Read the model definition and answer for the solid it produces. Units are mm, in the model's axes. A direction names the side the tool comes from. Round coordinates to 2 decimals unless told otherwise and drop trailing zeros. Order: outer loops, then holes, each group sorted by start corner. A loop starts at its lowest first (then second) coordinate and runs counter-clockwise, first axis right, second up. Notation, with made-up numbers: (24.25, -7) - (64.25, -7) arc R16 cw to (64.25, 6) - close; hole circle Ø1 at (80, -20.5). An arc over 180 degrees is marked (long way). Put each result on its own line as item: value. Start each with the question number.
Q1. Section C-C on x = -27.94 is taken. Give the vertices of the cut face in (y, z) (3 decimals).
Q2. Which of the six approach directions +Z, -Z, +X, -X, +Y, -Y give full straight-line access (tool end or side, diameter ignored) to faces 1 (the face through (-31.75, 4, 0)), 2 (the face through (0, 6.35, 0))?
Q3. Section A-A on z = -27.94 is taken. Give the vertices of the cut face in (x, y) (3 decimals).
Q4. For a pull along Z with two mould halves and no side action, classify faces 3 (the face through (-29.44, 3.88, -28.01)), 4 (the face through (14, 0, 0)), 5 (the face through (0, 4, -31.75)) as pulls with the +Z half, pulls with the -Z half, needs draft (parallel to the pull), parting line crosses it, or undercut.
Q5. This flat-tipped pin is pushed along its axis until it touches: pin 1 Ø7.5 at (x, z) = (-1.5, -3) entering from -Y. Where does it stop, or does it pass through?
Q6. Section D-D on z = 0 is taken. Give the vertices of the cut face in (x, y).
Q7. Find the intervals of material crossed by line 1 along X through (y, z) = (4, -27.94); line 2 along Z through (x, y) = (0, 4), in increasing order. Write a range as from..to.
Q8. Section B-B on y = 2 is taken. Give the vertices of the cut face in (x, z), then the cut area to 3 significant figures.
from build123d import *

# Parameters (mm, degrees)
SKETCH1_W                       = 63.5
SKETCH1_H                       = 63.5
BOSS_EXTRUDE1_DEPTH             = 7.62
F_3_0MM_DOWEL_HOLE1_D           = 3
F_3_0MM_DOWEL_HOLE1_DEPTH       = 7.62
F_3_0MM_DOWEL_HOLE1_CSINK_D     = 3.05
F_3_0MM_DOWEL_HOLE1_CSINK_ANGLE = 90
LPATTERN1_COUNT                 = 2
LPATTERN1_PITCH                 = 55.88
LPATTERN1_COUNT_DIR2            = 2
LPATTERN1_PITCH_DIR2            = 55.88
SKETCH6_R                       = 12.7
CUT_EXTRUDE1_DEPTH              = 6.35


with BuildPart() as part:
    # Sketch1 → Boss-Extrude1 (new body)
    with BuildSketch(Plane(origin=(0, 0, 0), x_dir=(1, 0, 0), z_dir=(0, 1, 0))):
        Rectangle(SKETCH1_W, SKETCH1_H)
    extrude(amount=BOSS_EXTRUDE1_DEPTH)

    # Ø3.0mm Dowel Hole1
    with Locations(Plane(origin=(0, 0, 0), x_dir=(-1, 0, 0), z_dir=(0, -1, 0))):
        with Locations((-27.94, -27.94)):
            f_3_0mm_dowel_hole1 = CounterSinkHole(F_3_0MM_DOWEL_HOLE1_D / 2, F_3_0MM_DOWEL_HOLE1_CSINK_D / 2, depth=F_3_0MM_DOWEL_HOLE1_DEPTH, counter_sink_angle=F_3_0MM_DOWEL_HOLE1_CSINK_ANGLE)

    # LPattern1: 3.0mm Dowel Hole1 2 × 2
    with Locations(*[(-j * LPATTERN1_PITCH_DIR2, 0, -i * LPATTERN1_PITCH) for i in range(LPATTERN1_COUNT) for j in range(LPATTERN1_COUNT_DIR2) if (i, j) != (0, 0)]):
        add(f_3_0mm_dowel_hole1, mode=Mode.SUBTRACT)

    # Sketch6 → Cut-Extrude1 (cut)
    with BuildSketch(Plane.XZ):
        Circle(SKETCH6_R)
    extrude(amount=-CUT_EXTRUDE1_DEPTH, mode=Mode.SUBTRACT)


solid = part.part
Findings:
1. outline: (0, -31.75) - (7.62, -31.75) - (7.62, -29.44) - (0.025, -29.44) - (0, -29.465) - close; (0, -26.415) - (0.025, -26.44) - (7.62, -26.44) - (7.62, 26.44) - (0.025, 26.44) - (0, 26.415) - close; (0, 29.465) - (0.025, 29.44) - (7.62, 29.44) - (7.62, 31.75) - (0, 31.75) - close
2. face 1: +Z, -Z, -X, +Y, -Y
2. face 2: -Y
3. outline: (-31.75, 0) - (-29.465, 0) - (-29.44, 0.025) - (-29.44, 7.62) - (-31.75, 7.62) - close; (-26.44, 0.025) - (-26.415, 0) - (26.415, 0) - (26.44, 0.025) - (26.44, 7.62) - (-26.44, 7.62) - close; (29.44, 0.025) - (29.465, 0) - (31.75, 0) - (31.75, 7.62) - (29.44, 7.62) - close
4. face 3: undercut
4. face 4: needs draft
4. face 5: pulls with the -Z half
5. pin 1: y = 6.35
6. outline: (-31.75, 0) - (-12.7, 0) - (-12.7, 6.35) - (12.7, 6.35) - (12.7, 0) - (31.75, 0) - (31.75, 7.62) - (-31.75, 7.62) - close
7. line 1: -31.75..-29.44, -26.44..26.44, 29.44..31.75
7. line 2: -31.75..-12.7, 12.7..31.75
8. outline: (-31.75, -31.75) - (31.75, -31.75) - (31.75, 31.75) - (-31.75, 31.75) - close; hole circle Ø3 at (-27.94, -27.94); hole circle Ø3 at (-27.94, 27.94); hole circle Ø25.4 at (0, 0); hole circle Ø3 at (27.94, -27.94); hole circle Ø3 at (27.94, 27.94)
8. area: 3,500 mm2
